Geometry: final body of the model. Coordinates: model frame, mm. Give positions to 0.01 mm unless a question says otherwise; leave off trailing zeros. Loops run counter-clockwise (first coordinate to the right, second up) from the corner with the lowest first, then second, coordinate; pieces in that order, holes last.
```python
from build123d import *

# Parameters (mm, degrees)
F0_W     = 121
F0_H     = 61.5
F1_DEPTH = 9
F2_R     = 2.726864
F2_R_2   = 3.05
F3_DEPTH = 10
F4_R     = 1.25
F5_DEPTH = 10
F6_R     = 1.65
F7_DEPTH = 10
F9_DEPTH = 125


with BuildPart() as f1:
    # F0 (on Top) → F1 (new body)
    with BuildSketch(Plane.XY):
        with Locations((-44.752393, 5.581188)):
            Rectangle(F0_W, F0_H)
    extrude(amount=-F1_DEPTH)

    # F2 (on face) → F3 (cut)
    with BuildSketch(Plane.XY):
        with Locations((-84.752393, 15.581188)):
            Circle(F2_R)
        with Locations((-84.752393, -4.418812)):
            Circle(F2_R_2)
        with Locations((-64.752393, 15.581188)):
            Circle(F2_R)
        with Locations((-64.752393, -4.418812)):
            Circle(F2_R_2)
        with Locations((-44.752393, 15.581188)):
            Circle(F2_R)
        with Locations((-44.752393, -4.418812)):
            Circle(F2_R_2)
        with Locations((-24.752393, 15.581188)):
            Circle(F2_R)
        with Locations((-24.752393, -4.418812)):
            Circle(F2_R_2)
        with Locations((-4.752393, 15.581188)):
            Circle(F2_R)
        with Locations((-4.752393, -4.418812)):
            Circle(F2_R_2)
    extrude(amount=-F3_DEPTH, mode=Mode.SUBTRACT)

    # F4 (on face) → F5 (cut)
    with BuildSketch(Plane(origin=(0, 0, -9), x_dir=(1, 0, 0), z_dir=(0, 0, -1))):
        with Locations((-97.252393, 17.168812)):
            Circle(F4_R)
        with Locations((-97.252393, -28.331188)):
            Circle(F4_R)
        with Locations((7.747607, 17.168812)):
            Circle(F4_R)
        with Locations((7.747607, -28.331188)):
            Circle(F4_R)
    extrude(amount=-F5_DEPTH, mode=Mode.SUBTRACT)

    # F6 (on face) → F7 (cut)
    with BuildSketch(Plane(origin=(0, 0, -9), x_dir=(1, 0, 0), z_dir=(0, 0, -1))):
        with Locations((-89.752393, -5.581188)):
            Circle(F6_R)
        with Locations((0.247607, -5.581188)):
            Circle(F6_R)
    extrude(amount=-F7_DEPTH, mode=Mode.SUBTRACT)

    # F8 (on face) → F9 (cut)
    with BuildSketch(Plane.YZ.offset(15.747607)):
        Polygon((-3.218812, 0), (-5.618812, 0), (-4.418812, -1.2), align=None)
        Polygon((16.781188, 0), (14.381188, 0), (15.581188, -1.2), align=None)
    extrude(amount=-F9_DEPTH, mode=Mode.SUBTRACT)


solid = f1.part
```
Q1. Material intervals for probe 1 along Y at (x, z) = (-63, -6.75); probe 2 along Y at (x, z) = (1.5, -1); probe 3 along X at (y, z) = (-18, -2.75), sorted ascending.
Q2. Section query A-A, the plane x = -24. Return loops of the section in (y, z).
Q3. Section query B-B, the plane z = -3.5. State how many separate pieces and enclosed holes the cut face has, and give its area (3 significant figures).
Q4. Mould query, pull axis X, two halves, no side actions, for faces 1 (the face through (-46, 36.331, -4)), 2 (the face through (-96.098, 28.81, -4.563)), 3 (the face through (-88.228, 6.213, -4.563)), 4 (the face through (15.748, 5, -4)). Classes: +X half, -X half, draft (parallel to the pull), parting line (faces both ways), or undercut.
Q5. Pin query (flat end, axial travel): pin 1 Ø3.5 at (x, y) = (-64.75, -4.42) entering from +Z; pin 2 Ø7 at (x, y) = (-24.75, -4.42) entering from +Z. Return the tip coordinate at first contact, or that it passes through.
Resolved:
1. probe 1: y = -25.17 to -6.92, -1.92 to 13.49, 17.67 to 36.33
1. probe 2: y = -25.17 to -4.62, -4.22 to 4.51, 6.66 to 15.38, 15.78 to 36.33
1. probe 3: x = -105.25 to -98.19, -96.32 to 6.81, 8.68 to 15.75
2. outline: (-25.17, -9) - (-7.37, -9) - (-7.37, 0) - (-25.17, 0) - close; (-1.46, -9) - (12.96, -9) - (12.96, 0) - (-1.46, 0) - close; (18.2, -9) - (36.33, -9) - (36.33, 0) - (18.2, 0) - close
3. separate pieces: 1
3. enclosed holes: 16
3. area: 7,140 mm2
4. face 1: draft
4. face 2: undercut
4. face 3: undercut
4. face 4: +X half
5. pin 1: passes through
5. pin 2: stops at z = 0
